For this review, take the finished solid that the model builds, in its own axes (mm). A direction names the side the tool comes from. Give positions to 0.01 mm unless a question says otherwise; leave off trailing zeros. Loops run counter-clockwise (first coordinate to the right, second up) from the corner with the lowest first, then second, coordinate; pieces in that order, holes last. Notation, with made-up numbers: (89, 23) - (108, 23) arc R37 ccw to (108, 62) - close; hole circle Ø8 at (55.5, 39.5). An arc over 180 degrees is marked (long way). Use CSV: the item, a comma, the result in double quotes. Start each with the question number.
1. Take a section at C-C on x = 11.5. Give the boundary of the cut face in (y, z).
2. Wall thickness on line 1 (X direction, y = -2, z = 15.5) (3 decimals); line 2 (Z direction, x = 26.9, y = -4.75) (3 decimals); line 3 (X direction, y = -6.75, z = 5): over which ranges is each line inside the solid? List them lowest first.
3. Mouldability with a two-part tool opening along X and no side actions: class faces 1 (the flat face through (27.64, -4.458, -16.805)), 2 (the flat face through (0, 1, 17.5)), 3 (the cylindrical face through (-27.033, -3.484, 16.516)) as pulls with the +X half, pulls with the -X half, needs draft (parallel to the pull), parting line crosses it, or undercut.
4. Take a section at D-D on z = 11. Give the boundary of the cut face in (x, y).
5. For pin 1 (10 mm diameter, centred on x = 6.5, z = 0, fed in from +Y); pin 2 (1.4 mm diameter, centred on y = -4, z = 16, fed in from +X); pin 3 (1.7 mm diameter, centred on y = -3, z = 0.5, fed in from -X), all flat-tipped, find the tip position at first contact; note any pin that passes through.
6. Take a section at A-A on y = -3. State how many separate pieces and enclosed holes the cut face has, plus the area to 3 significant figures.
7. For faces 4 (the flat face through (-26.14, -4.458, -16.793)), 5 (the flat face through (24.9, -4, 0)), 6 (the flat face through (-25.4, -4, 15)), list the 3-axis set-ups (+Z, -Z, +X, -X, +Y, -Y) from which the entire face can be reached by the end or side of a thin tool; tool diameter is ignored.
```python
from build123d import *

# Parameters (mm, degrees)
SKETCH1_W                          = 58.8
SKETCH1_H                          = 36
BOSS_EXTRUDE1_DEPTH                = 1.5
SKETCH1_3_W                        = 48
SKETCH1_3_H                        = 35
BOSS_EXTRUDE2_DEPTH                = 2.8
FILLET1_R                          = 1.5
BOSS_EXTRUDE3_START                = -1.5
BOSS_EXTRUDE3_DEPTH                = 6
M2_5X0_45_TAPPED_HOLE1_D           = 2.05
M2_5X0_45_TAPPED_HOLE1_CSINK_D     = 2.55
M2_5X0_45_TAPPED_HOLE1_CSINK_ANGLE = 60
SKETCH5_W                          = 44
SKETCH5_H                          = 34
CUT_EXTRUDE2_DEPTH                 = 0.1
MIRROR3_START                      = -1.5
MIRROR3_COPY_1_DEPTH               = 6
MIRROR3_COPY_2_D                   = 2.05
MIRROR3_COPY_2_CSINK_D             = 2.55
MIRROR3_COPY_2_CSINK_ANGLE         = 60
SKETCH9_W                          = 6
SKETCH9_H                          = 20
BOSS_EXTRUDE4_DEPTH                = 5.75


with BuildPart() as part:
    # Sketch1 → Boss-Extrude1 (new body)
    with BuildSketch(Plane(origin=(0, 0, 0), x_dir=(1, 0, 0), z_dir=(0, 1, 0))):
        Rectangle(SKETCH1_W, SKETCH1_H)
    extrude(amount=-BOSS_EXTRUDE1_DEPTH)

    # Sketch1<3> → Boss-Extrude2 (add)
    with BuildSketch(Plane(origin=(0, 0, 0), x_dir=(1, 0, 0), z_dir=(0, 1, 0))):
        Rectangle(SKETCH1_3_W, SKETCH1_3_H)
    extrude(amount=BOSS_EXTRUDE2_DEPTH)

    # Fillet1
    fillet1_edges = [part.edges().sort_by_distance(p)[0] for p in [
        (-29.4, -0.75, 18),
        (-29.4, -0.75, -18),
        (29.4, -0.75, -18),
        (29.4, -0.75, 18),
    ]]
    fillet(fillet1_edges, radius=FILLET1_R)

    # Sketch3 → Boss-Extrude3 (add)
    with BuildSketch(Plane(origin=(0, 0, 0), x_dir=(1, 0, 0), z_dir=(0, 1, 0)).offset(BOSS_EXTRUDE3_START)):
        Polygon((-26.9, 17.232050808), (-28.4, 16.366025404), (-28.4, 14.633974596), (-26.9, 13.767949192), (-25.4, 14.633974596), (-25.4, 16.366025404), align=None)
    boss_extrude3 = extrude(amount=-BOSS_EXTRUDE3_DEPTH)

    # M2.5x0.45 Tapped Hole1 (through all)
    with Locations(Plane(origin=(0, -7.5, 0), x_dir=(-1, 0, 0), z_dir=(0, -1, 0))):
        with Locations((26.9, 15.5)):
            m2_5x0_45_tapped_hole1 = CounterSinkHole(M2_5X0_45_TAPPED_HOLE1_D / 2, M2_5X0_45_TAPPED_HOLE1_CSINK_D / 2, counter_sink_angle=M2_5X0_45_TAPPED_HOLE1_CSINK_ANGLE)

    # Sketch5 → Cut-Extrude2 (cut)
    with BuildSketch(Plane(origin=(0, 2.8, 0), x_dir=(1, 0, 0), z_dir=(0, 1, 0))):
        with Locations((1.5, 0)):
            Rectangle(SKETCH5_W, SKETCH5_H)
    extrude(amount=-CUT_EXTRUDE2_DEPTH, mode=Mode.SUBTRACT)

    # Mirror2: Boss-Extrude3, M2.5x0.45 Tapped Hole1 across plane
    add(boss_extrude3.mirror(Plane.XY))
    add(m2_5x0_45_tapped_hole1.mirror(Plane.XY), mode=Mode.SUBTRACT)

    # Mirror3: Boss-Extrude3, M2.5x0.45 Tapped Hole1 across plane
    add(boss_extrude3.mirror(Plane(origin=(0, 0, 0), x_dir=(0, 0, 1), z_dir=(1, 0, 0))))
    add(m2_5x0_45_tapped_hole1.mirror(Plane(origin=(0, 0, 0), x_dir=(0, 0, 1), z_dir=(1, 0, 0))), mode=Mode.SUBTRACT)

    # Mirror3 copy 1 sketch → Mirror3 copy 1 (add)
    with BuildSketch(Plane(origin=(0, 0, 0), x_dir=(-1, 0, 0), z_dir=(0, 1, 0)).offset(MIRROR3_START)):
        Polygon((-26.9, 17.232050808), (-28.4, 16.366025404), (-28.4, 14.633974596), (-26.9, 13.767949192), (-25.4, 14.633974596), (-25.4, 16.366025404), align=None)
    extrude(amount=-MIRROR3_COPY_1_DEPTH)

    # Mirror3 copy 2 (through all)
    with Locations(Plane.XZ.offset(7.5)):
        with Locations((26.9, 15.5)):
            CounterSinkHole(MIRROR3_COPY_2_D / 2, MIRROR3_COPY_2_CSINK_D / 2, counter_sink_angle=MIRROR3_COPY_2_CSINK_ANGLE)

    # Sketch9 → Boss-Extrude4 (add)
    with BuildSketch(Plane.XZ.offset(1.5)):
        with Locations((21.9, 0)):
            Rectangle(SKETCH9_W, SKETCH9_H)
    extrude(amount=BOSS_EXTRUDE4_DEPTH)


solid = part.part
```
Check result:
1,outline,"(-1.5, -18) - (0, -18) - (0, -17.5) - (2.8, -17.5) - (2.8, -17) - (2.7, -17) - (2.7, 17) - (2.8, 17) - (2.8, 17.5) - (0, 17.5) - (0, 18) - (-1.5, 18) - close"
2,line 1,"x = -28.4 to -27.925, -25.875 to -25.4, 25.4 to 25.875, 27.925 to 28.4"
2,line 2,"z = -17.232 to -16.525, -14.475 to -13.768, 13.768 to 14.475, 16.525 to 17.232"
2,line 3,"x = 18.9 to 24.9"
3,face 1,"pulls with the +X half"
3,face 2,"needs draft"
3,face 3,"undercut"
4,outline,"(-29.4, -1.5) - (29.4, -1.5) - (29.4, 0) - (24, 0) - (24, 2.8) - (23.5, 2.8) - (23.5, 2.7) - (-20.5, 2.7) - (-20.5, 2.8) - (-24, 2.8) - (-24, 0) - (-29.4, 0) - close"
5,pin 1,"stops at y = 2.7"
5,pin 2,"stops at x = 28.4"
5,pin 3,"stops at x = 18.9"
6,separate pieces,"5"
6,enclosed holes,"4"
6,area,"138 mm²"
7,face 4,"-Z, -Y"
7,face 5,"+Z, -Z, +X, -Y"
7,face 6,"+Z, -Z, -Y"
